from build123d import *

# Parameters (mm, degrees)
SKETCH1_R               = 18.1
BOSS_EXTRUDE1_DEPTH     = 33.3
SKETCH2_R               = 1
CUT_EXTRUDE1_DEPTH      = 9.3
SKETCH3_R               = 2.45
CUT_EXTRUDE2_DEPTH      = 9.3
SKETCH4_W               = 4
SKETCH4_H               = 29.158742143
CUT_EXTRUDE3_DEPTH      = 66.637335137
CUT_EXTRUDE4_DEPTH      = 67.411402336
CUT_EXTRUDE4_DEPTH_BACK = 67.411402336
SKETCH5_R               = 1
SKETCH6_R               = 2.45
CUT_EXTRUDE5_DEPTH      = 22
BOSS_EXTRUDE2_DEPTH     = 5


with BuildPart() as part:
    # Sketch1 → Boss-Extrude1 (new body)
    with BuildSketch(Plane.XY):
        with BuildLine():
            ThreePointArc((26.098059899, 27.8276923), (-15.592298008, 44.914409405), (-12.023310526, 0))
            Line((-12.023310526, 0), (12.023310526, 0))
            ThreePointArc((12.023310526, 0), (21.360009365, 7.962102032), (26.098059899, 19.28110778))
            Line((26.098059899, 19.28110778), (26.098059899, 27.8276923))
        make_face()
        with Locations((0, 23.55440004)):
            Circle(SKETCH1_R, mode=Mode.SUBTRACT)
    extrude(amount=BOSS_EXTRUDE1_DEPTH)

    # Sketch2 → Cut-Extrude1 (cut)
    with BuildSketch(Plane.XZ):
        with Locations(Location((-7.5, 28.65, 0), (0, 0, 270))):
            Circle(SKETCH2_R)
        with Locations(Location((7.5, 28.65, 0), (0, 0, 270))):
            Circle(SKETCH2_R)
        with Locations(Location((-7.5, 4.65, 0), (0, 0, 270))):
            Circle(SKETCH2_R)
        with Locations(Location((7.5, 4.65, 0), (0, 0, 270))):
            Circle(SKETCH2_R)
    extrude(amount=-CUT_EXTRUDE1_DEPTH, mode=Mode.SUBTRACT)

    # Sketch3 → Cut-Extrude2 (cut)
    with BuildSketch(Plane(origin=(0, 4, 0), x_dir=(-1, 0, 0), z_dir=(0, -1, 0))):
        with Locations(Location((-7.5, -4.65, 0), (0, 0, 90))):
            Circle(SKETCH3_R)
        with Locations(Location((7.5, -4.65, 0), (0, 0, 90))):
            Circle(SKETCH3_R)
        with Locations(Location((-7.5, -28.65, 0), (0, 0, 90))):
            Circle(SKETCH3_R)
        with Locations(Location((7.5, -28.65, 0), (0, 0, 90))):
            Circle(SKETCH3_R)
    extrude(amount=-CUT_EXTRUDE2_DEPTH, mode=Mode.SUBTRACT)

    # Sketch4 → Cut-Extrude3 (cut, through all)
    with BuildSketch(Plane.XY.offset(33.3)):
        with Locations((0, 46.869056607)):
            Rectangle(SKETCH4_W, SKETCH4_H)
    extrude(amount=-CUT_EXTRUDE3_DEPTH, mode=Mode.SUBTRACT)

    # Sketch5 → Cut-Extrude4 (cut, two sides: drawn at the far end of the back side and taken through both)
    with BuildSketch(Plane.ZY.offset(-2).offset(-CUT_EXTRUDE4_DEPTH_BACK)):
        with Locations((6.15, 45.733914025)):
            Circle(SKETCH5_R)
        with Locations((27.15, 45.466040673)):
            Circle(SKETCH5_R)
    extrude(amount=CUT_EXTRUDE4_DEPTH + CUT_EXTRUDE4_DEPTH_BACK, mode=Mode.SUBTRACT)

    # Sketch6 → Cut-Extrude5 (cut)
    with BuildSketch(Plane.ZY.offset(-10)):
        with Locations((6.15, 45.733914025)):
            Circle(SKETCH6_R)
        with Locations((27.15, 45.466040673)):
            Circle(SKETCH6_R)
    cut_extrude5 = extrude(amount=-CUT_EXTRUDE5_DEPTH, mode=Mode.SUBTRACT)

    # Mirror1: Cut-Extrude5 across plane
    add(cut_extrude5.mirror(Plane(origin=(0, 0, 0), x_dir=(0, 0, 1), z_dir=(1, 0, 0))), mode=Mode.SUBTRACT)

    # Sketch7 → Boss-Extrude2 (add)
    with BuildSketch(Plane(origin=(0, 0, 33.3), x_dir=(-1, 0, 0), z_dir=(0, 0, -1))):
        with BuildLine():
            Line((-26.098059899, 19.28110778), (-26.098059899, 27.8276923))
            ThreePointArc((-26.098059899, 27.8276923), (-17.872880838, 43.046190307), (-2, 49.924264606))
            Line((-2, 49.924264606), (-2, 39.845441603))
            ThreePointArc((-2, 39.845441603), (0, 7.141050741), (2, 39.845441603))
            Line((2, 39.845441603), (2, 49.924264606))
            ThreePointArc((2, 49.924264606), (25.928196209, 28.760012261), (12.023310526, 0))
            Line((12.023310526, 0), (-12.023310526, 0))
            ThreePointArc((-12.023310526, 0), (-21.360009365, 7.962102032), (-26.098059899, 19.28110778))
        make_face()
    extrude(amount=-BOSS_EXTRUDE2_DEPTH)


solid = part.part
Can you work these out from the model? Positions are in its coordinate system, mm. A direction names the side the tool comes from. Round coordinates to 2 decimals unless told otherwise and drop trailing zeros. Write each loop counter-clockwise with the first axis right and the second up, starting at its lowest first coordinate (ties: lowest second). Pieces come first, ordered by that corner, then holes. Notation, with made-up numbers: (51.5, -13.75) -> (84.5, -13.75) arc R33 ccw to (84.5, 21.25) -> close; hole circle Ø5 at (-7.5, 21.25). An arc over 180 degrees is marked (long way). One line per question, with ' | ' between items. Start each with the question number.
1) On a 3-axis mill with a long thin cutter (end or side, diameter ignored), from which of +Z, -Z, +X, -X, +Y, -Y can I reach the whole of each face in a straight line? I mean faces 1 (the cylindrical face through (12.907, 43.286, 6.054)), 2 (the flat face through (6, 4, 29)), 3 (the cylindrical face through (-12.907, 43.286, 6.054)). Say none if no direction works.
2) I'm going to push flat-ended pins straight in: P1, Ø5, axis at x = 17, z = 19.5, coming from the +Y side; P2, Ø1, axis at x = -20.5, z = 24, coming from the -Y side; P3, Ø2.5, axis at y = 45.47, z = 27.15, coming from the -X side. Where does each tip first touch, or does it pass through?
3) I need wall thicknesses on line 1 (Z direction, x = -7.5, y = 5.3); line 2 (Z direction, x = -6, y = 4.5); line 3 (Z direction, x = -9, y = 37.5). Which ranges of each line are inside material? Lowest first, please. Write a range as [from, to].
4) Suppose I cut it at C-C on z = 34.5. Write out the boundary of the cut face in (x, y), then the cut area to 3 significant figures.
5) Suppose I cut it at D-D on x = 0. Write out the boundary of the cut face in (y, z).
6) Suppose I cut it at B-B on x = -7.5. Count the separate pieces of the cut face and the enclosed holes in it, then the cut area to 3 significant figures.
7) Suppose I cut it at A-A on y = 17.5. Write out the boundary of the cut face in (x, z), then the cut area to 3 significant figures.
8) If we mould it in two halves opening along Z, with no side actions, what happens to faces 4 (the flat face through (-4.1, 7.5, 33.3)), 5 (the flat face through (2, 45, 19)), 6 (the cylindrical face through (-7.46, 1.97, 29.65))? For each: released by +Z, released by -Z, zero draft, split by the parting line, or undercut.
Return value:
1) face 1: +X | face 2: none | face 3: -X
2) P1: stops at y = 45.67 | P2: stops at y = 6.25 | P3: stops at x = -10
3) line 1: z = [0, 2.2], [7.1, 26.2], [31.1, 38.3] | line 2: z = [0, 2.71], [6.59, 26.71], [30.59, 38.3] | line 3: z = [33.3, 38.3]
4) outline: (-12.02, 0) -> (12.02, 0) arc R26.45 ccw to (26.1, 19.28) -> (26.1, 27.83) arc R26.45 ccw to (2, 49.92) -> (2, 39.85) arc R16.41 cw (long way) to (-2, 39.85) -> (-2, 49.92) arc R26.45 ccw to start | area: 1,260 mm2
5) outline: (0, 0) -> (5.45, 0) -> (5.45, 33.3) -> (7.14, 33.3) -> (7.14, 38.3) -> (0, 38.3) -> close
6) separate pieces: 4 | enclosed holes: 2 | area: 578 mm2
7) outline: (-25.74, 0) -> (-17.06, 0) -> (-17.06, 33.3) -> (-15.26, 33.3) -> (-15.26, 38.3) -> (-25.74, 38.3) -> close; (15.26, 33.3) -> (17.06, 33.3) -> (17.06, 0) -> (25.74, 0) -> (25.74, 38.3) -> (15.26, 38.3) -> close | area: 683 mm2
8) face 4: released by -Z | face 5: zero draft | face 6: undercut
